from build123d import *

# Parameters (mm, degrees)
SCHIZZO1_W                   = 150
SCHIZZO1_H                   = 150
ESTRUSIONE_ESTRUSIONE1_DEPTH = 20
SCHIZZO2_W                   = 56
SCHIZZO2_H                   = 56
TAGLIO_ESTRUSIONE1_DEPTH     = 15
SCHIZZO3_R                   = 2.5
TAGLIO_ESTRUSIONE2_DEPTH     = 15
SMUSSO1_SIZE                 = 2
SCHIZZO4_R                   = 5
TAGLIO_ESTRUSIONE3_DEPTH     = 15
SMUSSO2_SIZE                 = 1


with BuildPart() as part:
    # Schizzo1 → Estrusione-Estrusione1 (new body)
    with BuildSketch(Plane(origin=(0, 0, 0), x_dir=(1, 0, 0), z_dir=(0, 1, 0))):
        Rectangle(SCHIZZO1_W, SCHIZZO1_H)
    extrude(amount=ESTRUSIONE_ESTRUSIONE1_DEPTH)

    # Schizzo2 → Taglio-Estrusione1 (cut)
    with BuildSketch(Plane(origin=(0, 20, 0), x_dir=(1, 0, 0), z_dir=(0, 1, 0))):
        Rectangle(SCHIZZO2_W, SCHIZZO2_H)
    extrude(amount=-TAGLIO_ESTRUSIONE1_DEPTH, mode=Mode.SUBTRACT)

    # Schizzo3 → Taglio-Estrusione2 (cut)
    with BuildSketch(Plane(origin=(0, 5, 0), x_dir=(1, 0, 0), z_dir=(0, 1, 0))):
        with Locations(Location((23.5, 23.5, 0), (0, 0, 270))):
            Circle(SCHIZZO3_R)
        with Locations(Location((-23.5, 23.5, 0), (0, 0, 270))):
            Circle(SCHIZZO3_R)
        with Locations(Location((-23.5, -23.5, 0), (0, 0, 270))):
            Circle(SCHIZZO3_R)
        with Locations(Location((23.5, -23.5, 0), (0, 0, 270))):
            Circle(SCHIZZO3_R)
    extrude(amount=-TAGLIO_ESTRUSIONE2_DEPTH, mode=Mode.SUBTRACT)

    # Smusso1
    smusso1_edges = [part.edges().sort_by_distance(p)[0] for p in [
        (28, 20, 0),
        (0, 20, -28),
        (-28, 20, 0),
        (0, 20, 28),
    ]]
    chamfer(smusso1_edges, length=SMUSSO1_SIZE)

    # Schizzo4 → Taglio-Estrusione3 (cut)
    with BuildSketch(Plane(origin=(0, 0, 0), x_dir=(-1, 0, 0), z_dir=(0, -1, 0))):
        with Locations(Location((60, -60, 0), (0, 0, 90))):
            Circle(SCHIZZO4_R)
        with Locations(Location((-60, -60, 0), (0, 0, 270))):
            Circle(SCHIZZO4_R)
        with Locations(Location((-60, 60, 0), (0, 0, 90))):
            Circle(SCHIZZO4_R)
        with Locations(Location((60, 60, 0), (0, 0, 270))):
            Circle(SCHIZZO4_R)
    extrude(amount=-TAGLIO_ESTRUSIONE3_DEPTH, mode=Mode.SUBTRACT)

    # Smusso2
    smusso2_edges = [part.edges().sort_by_distance(p)[0] for p in [
        (-60, 0, 65),
        (60, 0, 55),
        (60, 0, -55),
        (-60, 0, -65),
    ]]
    chamfer(smusso2_edges, length=SMUSSO2_SIZE)


solid = part.part
Could you check a few things on this model? Use its own coordinates, in mm. A direction names the side the tool comes from. Coordinates: 2 decimals unless noted, no trailing zeros. Order: outer loops, then holes, each group sorted by start corner. A loop starts at its lowest first (then second) coordinate and runs counter-clockwise, first axis right, second up. Notation, with made-up numbers: (58.5, 80) -> (90.5, 80) arc R23 cw to (90.5, 100) -> close; hole circle Ø1 at (49, 77). An arc over 180 degrees is marked (long way). One line per item, written item: value. Start each with the question number.
1) We'd pull the mould along Z, two halves only. Please class faces 4 (the flat face through (0, 12, 28)), 5 (the flat face through (-1, 10, 75)), 6 (the flat face through (75, 10, 1)): +Z half, -Z half, draft (parallel to the pull), parting line (faces both ways), or undercut.
2) Imagine slicing it at A-A on x = 23.5. List the corners of the cut face in (y, z) for me, plus the area to 3 significant figures.
3) If I drill on L1, parallel to X at y = 6, z = 60; L2, parallel to X at y = 3.55, z = 23.5; L3, parallel to Z at x = 25.5, y = 6.5, over which ranges is the centre line in solid material (lowest first)? Write a range as [from, to].
4) Which directions (+Z, -Z, +X, -X, +Y, -Y) give clear straight access to the entire face, cutting with the end or side of a thin tool? Please do faces 1 (the flat face through (-60, 15, -60)), 2 (the flat face through (0, 5, 0)), 3 (the cylindrical face through (-21.81, 2.54, 21.66)).
5) I'm going to push flat-ended pins straight in: pin 1 (5 mm diameter, centred on x = 60.5, z = 62.5, fed in from -Y); pin 2 (5 mm diameter, centred on x = -61, z = 60, fed in from -Y); pin 3 (12 mm diameter, centred on x = 8.5, z = 16, fed in from +Y). Where does each tip first touch, or does it pass through?
6) Imagine slicing it at D-D on z = 60. List the corners of the cut face in (x, y) for me, plus the area to 3 significant figures.
7) Imagine slicing it at B-B on z = 23.5. List the corners of the cut face in (x, y) for me, plus the area to 3 significant figures.
8) Imagine slicing it at C-C on y = 12. List the corners of the cut face in (x, z) for me.
Answer list:
1. face 4: undercut
1. face 5: +Z half
1. face 6: draft
2. outline: (0, -75) -> (20, -75) -> (20, -30) -> (18, -28) -> (5, -28) -> (5, -26) -> (0, -26) -> close; (0, -21) -> (5, -21) -> (5, 21) -> (0, 21) -> close; (0, 26) -> (5, 26) -> (5, 28) -> (18, 28) -> (20, 30) -> (20, 75) -> (0, 75) -> close
2. area: 2,110 mm2
3. L1: x = [-75, -65], [-55, 55], [65, 75]
3. L2: x = [-75, -26], [-21, 21], [26, 75]
3. L3: z = [-75, -28], [28, 75]
4. face 1: -Y
4. face 2: +Y
4. face 3: +Y, -Y
5. pin 1: stops at y = 0.95
5. pin 2: stops at y = 15
5. pin 3: stops at y = 5
6. outline: (-75, 0) -> (-66, 0) -> (-65, 1) -> (-65, 15) -> (-55, 15) -> (-55, 1) -> (-54, 0) -> (54, 0) -> (55, 1) -> (55, 15) -> (65, 15) -> (65, 1) -> (66, 0) -> (75, 0) -> (75, 20) -> (-75, 20) -> close
6. area: 2,700 mm2
7. outline: (-75, 0) -> (-26, 0) -> (-26, 5) -> (-28, 5) -> (-28, 18) -> (-30, 20) -> (-75, 20) -> close; (-21, 0) -> (21, 0) -> (21, 5) -> (-21, 5) -> close; (26, 0) -> (75, 0) -> (75, 20) -> (30, 20) -> (28, 18) -> (28, 5) -> (26, 5) -> close
7. area: 2,110 mm2
8. outline: (-75, -75) -> (75, -75) -> (75, 75) -> (-75, 75) -> close; hole circle Ø10 at (-60, -60); hole circle Ø10 at (-60, 60); hole (-28, -28) -> (28, -28) -> (28, 28) -> (-28, 28) -> close; hole circle Ø10 at (60, -60); hole circle Ø10 at (60, 60)
